Geometry check sheet. Reference: the model listing, model coordinates, mm. A direction names the side the tool comes from. Round coordinates to 2 decimals unless told otherwise and drop trailing zeros. Loops run counter-clockwise (first coordinate to the right, second up) from the corner with the lowest first, then second, coordinate; pieces in that order, holes last. Notation, with made-up numbers: (-11.75, 1.5) - (0.25, 1.5) arc R15 cw to (0.25, 26.5) - close; hole circle Ø1 at (-15, 63). An arc over 180 degrees is marked (long way). Write item = value, one per line.
```python
from build123d import *

# Parameters (mm, degrees)
F0_R     = 10
F1_DEPTH = 25.4
F3_DEPTH = 25.4
F4_DEPTH = 25.4
F5_SIZE  = 2.286


# Not quite as in the source:
# - the program builds the solid bodies; features that only make, move or delete a surface that nothing else refers to are left out


with BuildPart() as f1:
    # F0 (on Front) → F1 (new body)
    with BuildSketch(Plane.XZ):
        with BuildLine():
            ThreePointArc((3.7085113233, -24.7234088217), (18.9435052601, -16.313908436), (25, 0))
            ThreePointArc((25, 0), (18.9435052601, 16.313908436), (3.7085113233, 24.7234088217))
            ThreePointArc((3.7085113233, 24.7234088217), (-25, 0), (3.7085113233, -24.7234088217))
        make_face()
        Circle(F0_R, mode=Mode.SUBTRACT)
        with BuildLine():
            ThreePointArc((3.7085113233, 24.7234088217), (18.9435052601, 16.313908436), (25, 0))
            ThreePointArc((25, 0), (18.9435052601, -16.313908436), (3.7085113233, -24.7234088217))
            Line((3.7085113233, -24.7234088217), (53.1553289667, -17.3063861752))
            ThreePointArc((53.1553289667, -17.3063861752), (33.0593710404, 0), (53.1553289667, 17.3063861752))
            Line((53.1553289667, 17.3063861752), (3.7085113233, 24.7234088217))
        make_face()
        with BuildLine():
            ThreePointArc((68.0593710404, 0), (63.8198247225, 11.4197359052), (53.1553289667, 17.3063861752))
            ThreePointArc((53.1553289667, 17.3063861752), (33.0593710404, 0), (53.1553289667, -17.3063861752))
            ThreePointArc((53.1553289667, -17.3063861752), (63.8198247225, -11.4197359052), (68.0593710404, 0))
        make_face()
        with Locations((50.5593710404, 0)):
            Circle(F0_R, mode=Mode.SUBTRACT)
    extrude(amount=F1_DEPTH)

    # F0 (on Front) → F3 (join)
    with BuildSketch(Plane.XZ):
        with BuildLine():
            ThreePointArc((3.7085113233, -24.7234088217), (18.9435052601, -16.313908436), (25, 0))
            ThreePointArc((25, 0), (18.9435052601, 16.313908436), (3.7085113233, 24.7234088217))
            ThreePointArc((3.7085113233, 24.7234088217), (-25, 0), (3.7085113233, -24.7234088217))
        make_face()
        Circle(F0_R, mode=Mode.SUBTRACT)
        with BuildLine():
            ThreePointArc((68.0593710404, 0), (63.8198247225, 11.4197359052), (53.1553289667, 17.3063861752))
            ThreePointArc((53.1553289667, 17.3063861752), (33.0593710404, 0), (53.1553289667, -17.3063861752))
            ThreePointArc((53.1553289667, -17.3063861752), (63.8198247225, -11.4197359052), (68.0593710404, 0))
        make_face()
        with Locations((50.5593710404, 0)):
            Circle(F0_R, mode=Mode.SUBTRACT)
    extrude(amount=F3_DEPTH)

    # F0 (on Front) → F4 (join)
    with BuildSketch(Plane.XZ):
        with BuildLine():
            ThreePointArc((3.7085113233, -24.7234088217), (18.9435052601, -16.313908436), (25, 0))
            ThreePointArc((25, 0), (18.9435052601, 16.313908436), (3.7085113233, 24.7234088217))
            ThreePointArc((3.7085113233, 24.7234088217), (-25, 0), (3.7085113233, -24.7234088217))
        make_face()
        Circle(F0_R, mode=Mode.SUBTRACT)
        with BuildLine():
            ThreePointArc((68.0593710404, 0), (63.8198247225, 11.4197359052), (53.1553289667, 17.3063861752))
            ThreePointArc((53.1553289667, 17.3063861752), (33.0593710404, 0), (53.1553289667, -17.3063861752))
            ThreePointArc((53.1553289667, -17.3063861752), (63.8198247225, -11.4197359052), (68.0593710404, 0))
        make_face()
        with Locations((50.5593710404, 0)):
            Circle(F0_R, mode=Mode.SUBTRACT)
    extrude(amount=-F4_DEPTH)

    # F5
    f5_edges = [f1.edges().sort_by_distance(p)[0] for p in [
        (-10, 25.4, 0),
        (-25, 25.4, 0),
        (33.059371, 25.4, 0),
        (40.559371, 25.4, 0),
    ]]
    chamfer(f5_edges, length=F5_SIZE)


solid = f1.part
```
(1) Scan lines: L1, parallel to X at y = -13, z = -1.5; L2, parallel to Z at x = 0, y = 0; L3, parallel to Z at x = 63, y = 14.5. Record each from-to range of solid material in increasing order. Write a range as [from, to].
Answers follow:
L1 = [-24.95, -9.89], [9.89, 40.67], [60.45, 67.99]
L2 = [-25, -10], [10, 25]
L3 = [-12.31, 12.31]
(2) Gauge pin test, flat ends, axial feed: pin 1 (12 mm diameter, centred on y = 1.5, z = 11, fed in from +X); pin 2 (12 mm diameter, centred on y = -3.5, z = -19.5, fed in from +X); pin 3 (12 mm diameter, centred on x = 50.56, z = 0, fed in from +Y); pin 4 (3 mm diameter, centred on x = -3, z = -10, fed in from +Y). Record the tip position at first contact, or that the pin passes through.
Answers follow:
pin_1 = 67.33
pin_2 = 61.69
pin_3 = through
pin_4 = 25.05
(3) Section check B-B (x = 0). Enter the section's corners in (y, z).
Answers follow:
outline = (-25.4, -25) - (23.11, -25) - (25.4, -22.71) - (25.4, -12.29) - (23.11, -10) - (-25.4, -10) - close; (-25.4, 10) - (23.11, 10) - (25.4, 12.29) - (25.4, 22.71) - (23.11, 25) - (-25.4, 25) - close
(4) Section check C-C (y = -3.5). Enter the section's corners in (x, z).
Answers follow:
outline = (3.71, -24.72) - (53.16, -17.31) arc R17.5 ccw to (53.16, 17.31) - (3.71, 24.72) arc R25 ccw (long way) to start; hole circle Ø20 at (0, 0); hole circle Ø20 at (50.56, 0)
(5) Set-up check for faces 5 (the cylindrical face through (-2.17, -0.8, -9.76)), 6 (the flat face through (30, 0, -2)): record each of +Z, -Z, +X, -X, +Y, -Y from which the full face is reachable in a straight line by a thin tool's end or side.
Answers follow:
face_5 = +Y, -Y
face_6 = +Y
(6) Section check A-A (y = 17.5). Enter the section's corners in (x, z).
Answers follow:
outline = circle Ø50 at (0, 0); circle Ø35 at (50.56, 0); hole circle Ø20 at (0, 0); hole circle Ø20 at (50.56, 0)
(7) Mould release check, pull along Z, two halves, no side actions. Record for faces 1 (the flat face through (28.086, -12.522, -21.067)), 2 (the conical face through (42.536, 23.225, -6.152)), 3 (the flat face through (10, 25.4, -10)), 4 (the cylindrical face through (40.57, -0.8, 0.44)): pulls with the +Z half, pulls with the -Z half, needs draft (parallel to the pull), parting line crosses it, or undercut.
Answers follow:
face_1 = pulls with the -Z half
face_2 = undercut
face_3 = needs draft
face_4 = undercut
(8) Section check D-D (z = -6). State how many separate pieces and enclosed holes the cut face has, then the cut area to 3 significant figures.
Answers follow:
separate_pieces = 3
enclosed_holes = 0
area = 2,740 mm²
